from build123d import *

# Parameters (mm, degrees)
ESQUISSE4_W                    = 88
ESQUISSE4_H                    = 58
BOSS_EXTRU_3_DEPTH             = 3.3
ESQUISSE5_W                    = 8
ESQUISSE5_H                    = 3.3
BOSS_EXTRU_6_DEPTH             = 3.3
R_P_TITION_LIN_AIRE2_COUNT     = 3
R_P_TITION_LIN_AIRE2_PITCH     = 16
R_P_TITION_LIN_AIRE2_COL_COUNT = 3
R_P_TITION_LIN_AIRE2_COL_PITCH = 16
SYM_TRIE1_COPY_1_SKETCH_W      = 8
SYM_TRIE1_COPY_1_SKETCH_H      = 3.3
SYM_TRIE1_COPY_1_DEPTH         = 3.3
SYM_TRIE1_COPY_2_SKETCH_W      = 8
SYM_TRIE1_COPY_2_SKETCH_H      = 3.3
SYM_TRIE1_COPY_2_DEPTH         = 3.3
SYM_TRIE1_COPY_3_SKETCH_W      = 8
SYM_TRIE1_COPY_3_SKETCH_H      = 3.3
SYM_TRIE1_COPY_3_DEPTH         = 3.3
SYM_TRIE1_COPY_4_SKETCH_W      = 8
SYM_TRIE1_COPY_4_SKETCH_H      = 3.3
SYM_TRIE1_COPY_4_DEPTH         = 3.3
ESQUISSE6_W                    = 3.3
ESQUISSE6_H                    = 8
BOSS_EXTRU_7_DEPTH             = 3.3
R_P_TITION_LIN_AIRE3_COUNT     = 2
R_P_TITION_LIN_AIRE3_PITCH     = 16
R_P_TITION_LIN_AIRE3_COL_COUNT = 2
R_P_TITION_LIN_AIRE3_COL_PITCH = 16
SYM_TRIE2_COPY_1_SKETCH_W      = 3.3
SYM_TRIE2_COPY_1_SKETCH_H      = 8
SYM_TRIE2_COPY_1_DEPTH         = 3.3
SYM_TRIE2_COPY_2_SKETCH_W      = 3.3
SYM_TRIE2_COPY_2_SKETCH_H      = 8
SYM_TRIE2_COPY_2_DEPTH         = 3.3
ESQUISSE7_R                    = 2.5
ESQUISSE7_W                    = 61
ESQUISSE7_H                    = 48
ENL_V_MAT_EXTRU_1_DEPTH        = 1
ENL_V_MAT_EXTRU_1_DEPTH_BACK   = 4.3


with BuildPart() as part:
    # Esquisse4 → Boss.-Extru.3 (new body)
    with BuildSketch(Plane(origin=(0, 0, 0), x_dir=(1, 0, 0), z_dir=(0, 1, 0))):
        Rectangle(ESQUISSE4_W, ESQUISSE4_H)
    extrude(amount=BOSS_EXTRU_3_DEPTH)

    # Esquisse5 → Boss.-Extru.6 (add)
    with BuildSketch(Plane.XZ):
        with Locations((0, 30.65)):
            Rectangle(ESQUISSE5_W, ESQUISSE5_H)
    boss_extru_6 = extrude(amount=-BOSS_EXTRU_6_DEPTH)

    # Répétition linéaire2: Boss.-Extru.6 ×3
    with Locations(*[(-i * R_P_TITION_LIN_AIRE2_PITCH, 0, 0) for i in range(1, R_P_TITION_LIN_AIRE2_COUNT)]):
        add(boss_extru_6)

    # Répétition linéaire2 col: Boss.-Extru.6 ×3
    with Locations(*[(i * R_P_TITION_LIN_AIRE2_COL_PITCH, 0, 0) for i in range(1, R_P_TITION_LIN_AIRE2_COL_COUNT)]):
        add(boss_extru_6)

    # Symétrie1: Boss.-Extru.6 across plane
    add(boss_extru_6.mirror(Plane.XY))

    # Symétrie1 copy 1 sketch → Symétrie1 copy 1 (add)
    with BuildSketch(Plane(origin=(-16, 0, 0), x_dir=(1, 0, 0), z_dir=(0, -1, 0))):
        with Locations((0, -30.65)):
            Rectangle(SYM_TRIE1_COPY_1_SKETCH_W, SYM_TRIE1_COPY_1_SKETCH_H)
    extrude(amount=-SYM_TRIE1_COPY_1_DEPTH)

    # Symétrie1 copy 2 sketch → Symétrie1 copy 2 (add)
    with BuildSketch(Plane(origin=(-32, 0, 0), x_dir=(1, 0, 0), z_dir=(0, -1, 0))):
        with Locations((0, -30.65)):
            Rectangle(SYM_TRIE1_COPY_2_SKETCH_W, SYM_TRIE1_COPY_2_SKETCH_H)
    extrude(amount=-SYM_TRIE1_COPY_2_DEPTH)

    # Symétrie1 copy 3 sketch → Symétrie1 copy 3 (add)
    with BuildSketch(Plane(origin=(16, 0, 0), x_dir=(1, 0, 0), z_dir=(0, -1, 0))):
        with Locations((0, -30.65)):
            Rectangle(SYM_TRIE1_COPY_3_SKETCH_W, SYM_TRIE1_COPY_3_SKETCH_H)
    extrude(amount=-SYM_TRIE1_COPY_3_DEPTH)

    # Symétrie1 copy 4 sketch → Symétrie1 copy 4 (add)
    with BuildSketch(Plane(origin=(32, 0, 0), x_dir=(1, 0, 0), z_dir=(0, -1, 0))):
        with Locations((0, -30.65)):
            Rectangle(SYM_TRIE1_COPY_4_SKETCH_W, SYM_TRIE1_COPY_4_SKETCH_H)
    extrude(amount=-SYM_TRIE1_COPY_4_DEPTH)

    # Esquisse6 → Boss.-Extru.7 (add)
    with BuildSketch(Plane.XZ):
        with Locations((-45.65, 0)):
            Rectangle(ESQUISSE6_W, ESQUISSE6_H)
    boss_extru_7 = extrude(amount=-BOSS_EXTRU_7_DEPTH)

    # Répétition linéaire3: Boss.-Extru.7 ×2
    with Locations(*[(0, 0, i * R_P_TITION_LIN_AIRE3_PITCH) for i in range(1, R_P_TITION_LIN_AIRE3_COUNT)]):
        add(boss_extru_7)

    # Répétition linéaire3 col: Boss.-Extru.7 ×2
    with Locations(*[(0, 0, -i * R_P_TITION_LIN_AIRE3_COL_PITCH) for i in range(1, R_P_TITION_LIN_AIRE3_COL_COUNT)]):
        add(boss_extru_7)

    # Symétrie2: Boss.-Extru.7 across plane
    add(boss_extru_7.mirror(Plane(origin=(0, 0, 0), x_dir=(0, 0, 1), z_dir=(1, 0, 0))))

    # Symétrie2 copy 1 sketch → Symétrie2 copy 1 (add)
    with BuildSketch(Plane(origin=(0, 0, 16), x_dir=(-1, 0, 0), z_dir=(0, -1, 0))):
        with Locations((-45.65, 0)):
            Rectangle(SYM_TRIE2_COPY_1_SKETCH_W, SYM_TRIE2_COPY_1_SKETCH_H)
    extrude(amount=-SYM_TRIE2_COPY_1_DEPTH)

    # Symétrie2 copy 2 sketch → Symétrie2 copy 2 (add)
    with BuildSketch(Plane(origin=(0, 0, -16), x_dir=(-1, 0, 0), z_dir=(0, -1, 0))):
        with Locations((-45.65, 0)):
            Rectangle(SYM_TRIE2_COPY_2_SKETCH_W, SYM_TRIE2_COPY_2_SKETCH_H)
    extrude(amount=-SYM_TRIE2_COPY_2_DEPTH)

    # Esquisse7 → Enlèv. mat.-Extru.1 (cut, two sides)
    with BuildSketch(Plane.XZ) as enl_v_mat_extru_1_sk:
        with Locations((35, -26.5)):
            Circle(ESQUISSE7_R)
        with Locations((-6.5, 3)):
            Rectangle(ESQUISSE7_W, ESQUISSE7_H)
    extrude(amount=ENL_V_MAT_EXTRU_1_DEPTH, mode=Mode.SUBTRACT)
    extrude(enl_v_mat_extru_1_sk.sketch, amount=-ENL_V_MAT_EXTRU_1_DEPTH_BACK, mode=Mode.SUBTRACT)


solid = part.part
Read the model definition and answer for the solid it produces. Units are mm, in the model's axes. A direction names the side the tool comes from. Round coordinates to 2 decimals unless told otherwise and drop trailing zeros. Write each loop counter-clockwise with the first axis right and the second up, starting at its lowest first coordinate (ties: lowest second). Pieces come first, ordered by that corner, then holes. Notation, with made-up numbers: (-33, 20) - (-23, 20) arc R27 ccw to (-23, 47) - close; hole circle Ø9 at (28.25, 41). An arc over 180 degrees is marked (long way). One line per question, with ' | ' between items. Start each with the question number.
1. Each of these flat-tipped pins is pushed along its axis until it touches: pin 1 (1 mm diameter, centred on x = 9, y = 2, fed in from +Z); pin 2 (1.6 mm diameter, centred on y = 2.5, z = 5.5, fed in from -X); pin 3 (1 mm diameter, centred on y = 1.5, z = -31, fed in from +X). Where does it stop, or does it pass through?
2. Section A-A (x = 35) is taken. Determine the outline of the cut face in (y, z), and give its area (3 significant figures).
3. For faces 1 (the face through (28, 2, 31)), 2 (the face through (-8, 2, -29)), 3 (the face through (-36, 2, -31)), determine the directions among +Z, -Z, +X, -X, +Y, -Y from which every point of the face is accessible in a straight line to the end or side of a thin tool.
4. Find the intervals of material crossed by probe 1 along Z at (x, y) = (-11, 2.65); probe 2 along Z at (x, y) = (35, 1.6); probe 3 along X at (y, z) = (1.7, 25.5), in increasing order. Write a range as [from, to].
5. For a pull along Z with two mould halves and no side action, classify faces 4 (the face through (-46, 2, -4)), 5 (the face through (46, 2, -12)), 6 (the face through (-47.3, 2, -16)), 7 (the face through (-46, 2, 20)) as +Z half, -Z half, draft (parallel to the pull), parting line (faces both ways), or undercut.
6. Section C-C (y = 2.05) is taken. Give the number of separate pieces and of enclosed holes in the cut face, and give its area (3 significant figures).
7. Section B-B (z = -19) is taken. Determine the outline of the cut face in (x, y).
Filled in:
1) pin 1: z = 29 | pin 2: x = -44 | pin 3: x = 36
2) outline: (0, -32.3) - (3.3, -32.3) - (3.3, -29) - (0, -29) - close; (0, -24) - (3.3, -24) - (3.3, 32.3) - (0, 32.3) - close | area: 197 mm²
3) face 1: +Z, +Y, -Y | face 2: -Z, +Y, -Y | face 3: -Z, -X, +Y, -Y
4) probe 1: [-29, -21], [27, 29] | probe 2: [-32.3, -29], [-24, 32.3] | probe 3: [-44, -37], [24, 44]
5) face 4: undercut | face 5: undercut | face 6: draft | face 7: +Z half
6) separate pieces: 1 | enclosed holes: 2 | area: 2,580 mm²
7) outline: (-47.3, 0) - (-37, 0) - (-37, 3.3) - (-47.3, 3.3) - close; (24, 0) - (47.3, 0) - (47.3, 3.3) - (24, 3.3) - close
